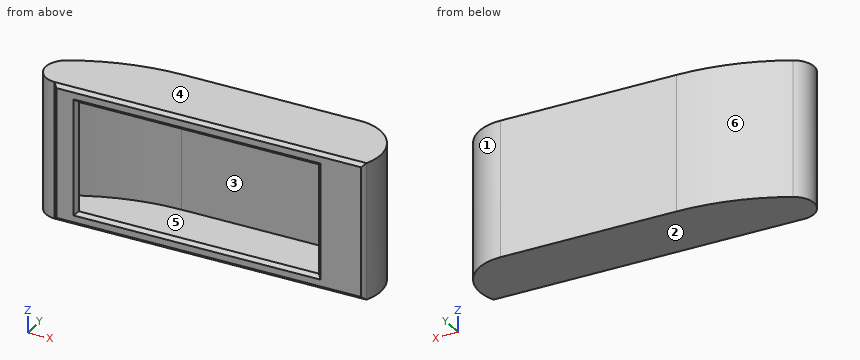
```python
from build123d import *

# Parameters (mm, degrees)
BOSS_EXTRUDE1_DEPTH = 38
BOSS_EXTRUDE2_START = 1
BOSS_EXTRUDE2_DEPTH = 1
SKETCH3_W           = 90.179925192
SKETCH3_H           = 40
SKETCH3_W_2         = 69.416494059
SKETCH3_H_2         = 32
BOSS_EXTRUDE3_DEPTH = 1
CHAMFER1_SIZE       = 1


with BuildPart() as part:
    # Sketch1 → Boss-Extrude1 (new body)
    with BuildSketch(Plane.XY):
        with BuildLine():
            Line((66.52, 14.5), (15.54, 14.5))
            ThreePointArc((15.54, 14.5), (0.223169493, 12.66316181), (-14.225037528, 7.256815055))
            ThreePointArc((-14.225037528, 7.256815055), (-17.376400179, 0.546177113), (-11.711514098, -4.236375954))
            Line((-11.711514098, -4.236375954), (-6.590403043, -4.236765961))
            Line((-6.590403043, -4.236765961), (-6.590326886, -3.236765964))
            Line((-6.590326886, -3.236765964), (-11.687025279, -3.236377816))
            ThreePointArc((-11.687025279, -3.236377816), (-16.401861513, 0.77072863), (-13.765555848, 6.368627808))
            ThreePointArc((-13.765555848, 6.368627808), (0.459614785, 11.691517006), (15.54, 13.5))
            Line((15.54, 13.5), (66.52, 13.5))
            ThreePointArc((66.52, 13.5), (76.617843982, 8.130760845), (77.812974461, -3.243193847))
            Line((77.812974461, -3.243193847), (72.705055873, -3.242804844))
            Line((72.705055873, -3.242804844), (72.704979716, -4.242804841))
            Line((72.704979716, -4.242804841), (78.468410832, -4.243243765))
            ThreePointArc((78.468410832, -4.243243765), (77.633884428, 8.404811863), (66.52, 14.5))
        make_face()
    extrude(amount=BOSS_EXTRUDE1_DEPTH)

    # Sketch2 → Boss-Extrude2 (add)
    with BuildSketch(Plane(origin=(0, 0, 0), x_dir=(-1, 0, 0), z_dir=(0, 0, -1)).offset(BOSS_EXTRUDE2_START)):
        with BuildLine():
            Line((-72.704979716, -4.242804841), (6.590403043, -4.236765961))
            Line((6.590403043, -4.236765961), (11.711514098, -4.236375954))
            ThreePointArc((11.711514098, -4.236375954), (17.376400179, 0.546177113), (14.225037528, 7.256815055))
            ThreePointArc((14.225037528, 7.256815055), (-0.223169493, 12.66316181), (-15.54, 14.5))
            Line((-15.54, 14.5), (-66.52, 14.5))
            ThreePointArc((-66.52, 14.5), (-77.633884428, 8.404811863), (-78.468410832, -4.243243765))
            Line((-78.468410832, -4.243243765), (-72.704979716, -4.242804841))
        make_face()
    boss_extrude2 = extrude(amount=-BOSS_EXTRUDE2_DEPTH)

    # Mirror1: Boss-Extrude2 across plane
    add(boss_extrude2.mirror(Plane.XY.offset(19)))

    # Sketch3 → Boss-Extrude3 (add)
    with BuildSketch(Plane(origin=(-0.000322697, -4.23726784, 0), x_dir=(0.9999999971000731, -7.615677136513779e-05, 0), z_dir=(-7.615677136513779e-05, -0.9999999971000731, 0))):
        with Locations((33.378771161, 19)):
            Rectangle(SKETCH3_W, SKETCH3_H)
        with Locations((29.997055594, 19)):
            Rectangle(SKETCH3_W_2, SKETCH3_H_2, mode=Mode.SUBTRACT)
    extrude(amount=BOSS_EXTRUDE3_DEPTH)

    # Chamfer1
    chamfer1_edges = [part.edges().sort_by_distance(p)[0] for p in [
        (-11.711590255, -5.236375951, 19),
        (-4.711590275, -5.236909048, 19),
        (29.996656654, -5.239552316, 3),
        (29.996656654, -5.239552316, 35),
        (64.704903583, -5.242195584, 19),
        (78.468334676, -5.243243763, 19),
        (33.37837221, -5.239809857, 39),
        (33.37837221, -5.239809857, -1),
    ]]
    chamfer(chamfer1_edges, length=CHAMFER1_SIZE - 0.0001)  # a hair under: the kernel refuses the full size


solid = part.part
```
The model under review builds one solid part; all positions refer to its coordinate system, in mm. Face numbers are marked on the shaded views. A direction names the side the tool comes from. Round coordinates to 2 decimals unless told otherwise and drop trailing zeros. Loops run counter-clockwise (first coordinate to the right, second up) from the corner with the lowest first, then second, coordinate; pieces in that order, holes last. Notation, with made-up numbers: M 35.25,-32.75 L 60.25,-32.75 A9 cw 60.25,-22.75 Z; hole C -21.5,15.25 d4. An arc over 180 degrees is marked long. Put each result on its own line as item: value.
Q1. For pin 1 (8 mm diameter, centred on x = 4.5, z = 26, fed in from -Y); pin 2 (0.5 mm diameter, centred on y = -3.5, z = 18.5, fed in from -X); pin 3 (0.5 mm diameter, centred on y = -3.5, z = 22.5, fed in from +X), all flat-tipped, find the tip position at first contact; note any pin that passes through.
Result set:
pin 1: stops at y = 11.7
pin 2: stops at x = -14.76
pin 3: stops at x = 78.88
Q2. Mouldability with a two-part tool opening along Z and no side actions: class the marked faces 1, 2, 3 and 4 as released by +Z, released by -Z, zero draft, split by the parting line, or undercut.
Result set:
face 1: zero draft
face 2: released by -Z
face 3: undercut
face 4: released by +Z
Q3. To check wall thickness, follow L1, parallel to Z at x = 32, y = 2; L2, parallel to X at y = 1.5, z = 35.5; L3, parallel to X at y = 2.5, z = 35. State the ranges of each line that lie inside material, in increasing order.
Result set:
L1: z = -1 to 0, 38 to 39
L2: x = -17.51 to -16.51, 78.7 to 79.7
L3: x = -17.48 to -16.48, 78.64 to 79.65
Q4. Machinability: for the marked faces 5 and 6, which of the approach directions +Z, -Z, +X, -X, +Y, -Y give a long, thin tool a straight path to every point of the face, cutting with its end or side? Answer none if there is none.
Result set:
face 5: none
face 6: +Z, -Z, -X, +Y
Q5. Consider section B-B, the plane x = 70.5. Give the boundary of the cut face in (y, z).
Result set:
outline: M -5.24,0 L -4.24,-1 L 13.88,-1 L 13.88,39 L -4.24,39 L -5.24,38 Z; hole M -4.24,0 L 12.83,0 L 12.83,38 L -4.24,38 Z
Q6. Consider section C-C, the plane y = 12. Give the boundary of the cut face in (x, z), then the cut area to 3 significant figures.
Result set:
outline: M -2.28,-1 L 74.24,-1 L 74.24,39 L -2.28,39 Z; hole M 1.79,0 L 72.38,0 L 72.38,38 L 1.79,38 Z
area: 379 mm²
